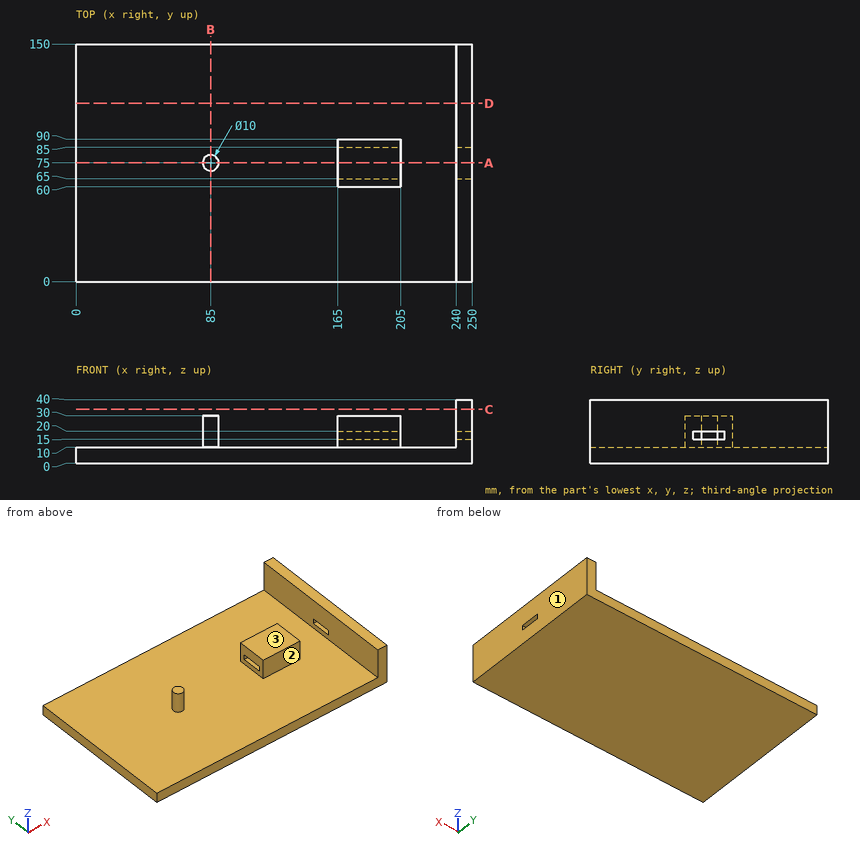
Could you check a few things on this drawing? It's one solid part, dimensions in mm from its lowest x, y, z. A direction names the side the tool comes from. Coordinates: 2 decimals unless noted, no trailing zeros. Loops run counter-clockwise (first coordinate to the right, second up) from the corner with the lowest first, then second, coordinate; pieces in that order, holes last. Notation, with made-up numbers: (79.5, 53) - (90.5, 53) arc R13 cw to (90.5, 76) - close; hole circle Ø10 at (39.5, 87.5). An arc over 180 degrees is marked (long way). Answer as a JSON object with one key per item and string values. Group by question number.
Item 1: If I drill on L1, parallel to X at y = 69, z = 11.5; L2, parallel to Z at x = 192, y = 73.5; L3, parallel to Z at x = 144, y = 22, over which ranges is the centre line in solid material (lowest first)? Write a range as from..to.
Item 2: For pin 1 (12 mm diameter, centred on x = 66, y = 48.5, fed in from +Z); pin 2 (8 mm diameter, centred on x = 85.5, y = 76.5, fed in from +Z); pin 3 (2.5 mm diameter, centred on x = 192.5, z = 17.5, fed in from -Y), each with a flat end and sliding along its axis, tell me the tip position at first contact or that it passes through.
Item 3: If we section it at C-C (z = 34): List the corners of the cut face in (x, y) for me, plus the area to 3 significant figures.
Item 4: If we section it at D-D (y = 112.5): List the corners of the cut face in (x, z) for me.
Item 5: If we section it at B-B (x = 85): List the corners of the cut face in (y, z) for me, plus the area to 3 significant figures.
Item 6: On a 3-axis mill with a long thin cutter (end or side, diameter ignored), from which of +Z, -Z, +X, -X, +Y, -Y can I reach the whole of each face in a straight line? I mean the marked faces 1, 2 and 3. Say none if no direction works.
Item 7: If we section it at A-A (y = 75): List the corners of the cut face in (x, z) for me, plus the area to 3 significant figures.
Returned:
{
 "1": {"L1": "x = 165..205, 240..250", "L2": "z = 0..15, 20..30", "L3": "z = 0..10"},
 "2": {"pin 1": "stops at z = 10", "pin 2": "stops at z = 30", "pin 3": "stops at y = 60"},
 "3": {"outline": "(240, 0) - (250, 0) - (250, 150) - (240, 150) - close", "area": "1,500 mm²"},
 "4": {"outline": "(0, 0) - (250, 0) - (250, 40) - (240, 40) - (240, 10) - (0, 10) - close"},
 "5": {"outline": "(0, 0) - (150, 0) - (150, 10) - (80, 10) - (80, 30) - (70, 30) - (70, 10) - (0, 10) - close", "area": "1,700 mm²"},
 "6": {"face 1": "+Z, -Z, +X, +Y, -Y", "face 2": "+Z, -X, -Y", "face 3": "+Z, -X, +Y, -Y"},
 "7": {"outline": "(0, 0) - (250, 0) - (250, 15) - (240, 15) - (240, 10) - (205, 10) - (205, 15) - (165, 15) - (165, 10) - (90, 10) - (90, 30) - (80, 30) - (80, 10) - (0, 10) - close; (165, 20) - (205, 20) - (205, 30) - (165, 30) - close; (240, 20) - (250, 20) - (250, 40) - (240, 40) - close", "area": "3,550 mm²"}
}
